Check sheet for the modelled part. Datum: model origin and axes. Units: mm. A direction names the side the tool comes from. Give positions to 0.01 mm unless a question says otherwise; leave off trailing zeros. Order: outer loops, then holes, each group sorted by start corner. A loop starts at its lowest first (then second) coordinate and runs counter-clockwise, first axis right, second up. Notation, with made-up numbers: (78.5, -18.75) -> (82.5, -18.75) arc R24 ccw to (82.5, -1.75) -> close; hole circle Ø8 at (28, 83.25). An arc over 180 degrees is marked (long way). Answer in a Markdown table with one row per item. Add a question column.
(1) Go/stop test with flat-tipped pins: pin 1 (1.5 mm diameter, centred on x = -1.5, z = -3.5, fed in from +Y); pin 2 (1 mm diameter, centred on x = 0.5, y = 1, fed in from -Z); pin 3 (0.6 mm diameter, centred on x = 3.5, z = 2, fed in from +Y); pin 4 (2 mm diameter, centred on x = 12, z = 10.5, fed in from -Y) (1 decimal). Record where each tip stops, or that it passes through.
(2) Cross-section at B-B (y = -2.5). Record the cut outline in (x, z) (1 decimal).
(3) Cross-section at A-A (x = -13). Record the cut outline in (y, z).
(4) Set-up check for faces 4 (the face through (-3.7, 1.295, 1.6)), 5 (the face through (16.66, 0.98, -0.11)): record each of +Z, -Z, +X, -X, +Y, -Y from which the full face is reachable in a straight line by a thin tool's end or side.
(5) Release check for a two-part mould opening along X. For faces 1 (the face through (1, -3.81, -3)), 2 (the face through (-2.8, 1.78, -2.8)), 3 (the face through (-11.182, 0.952, 2.915)) record: released by +X, released by -X, zero draft, split by the parting line, or undercut.
(6) Thickness scan on L1, parallel to Z at x = 0, y = 0.5; L2, parallel to Z at x = -7, y = 0.5; L3, parallel to X at y = -3.1, z = 0. Record the ranges inside material, lowest first. Write a range as [from, to].
```python
from build123d import *

# Parameters (mm, degrees)
EXTRUDE4_DEPTH          = 1.9304
SKETCH2_R               = 0.6604
CUT_EXTRUDE1_DEPTH      = 19.722050478
CIRPATTERN4_COUNT       = 6
SKETCH3_R               = 1.397
CUT_EXTRUDE2_DEPTH      = 12.7
CUT_EXTRUDE2_DEPTH_BACK = 12.7
SKETCH4_R               = 4.445
CUT_EXTRUDE3_DEPTH      = 0.635
SKETCH5_R               = 3.4925
SKETCH5_R_2             = 3.175
EXTRUDE5_DEPTH          = 1.143
RIB10_REACH             = 26.438
SKETCH8_WALL_W          = 52.220152264
SKETCH8_WALL_H          = 0.381
CIRPATTERN5_COUNT       = 8
SKETCH9_R               = 0.79375
CUT_EXTRUDE4_DEPTH      = 25.392925761
CIRPATTERN6_COUNT       = 6
SKETCH10_R              = 5.08
EXTRUDE6_DEPTH          = 0.762
FILLET2_R               = 0.508
SKETCH11_R              = 4.064
EXTRUDE7_DEPTH          = 3.048
FILLET3_R               = 0.889
SKETCH12_R              = 2.8575
CUT_EXTRUDE5_DEPTH      = 3.429
SKETCH14_R              = 1.397
CUT_EXTRUDE6_DEPTH      = 25.557003564
SKETCH15_R              = 0.3175
CUT_EXTRUDE7_DEPTH      = 25.984806887
CIRPATTERN7_COUNT       = 6


with BuildPart() as part:
    # Sketch1 → Extrude4 (new body)
    with BuildSketch(Plane(origin=(0, 0, 0), x_dir=(1, 0, 0), z_dir=(0, 1, 0))):
        with BuildLine():
            Line((5.775220615, -3.829827046), (0, 0))
            Line((0, 0), (5.775220615, 3.829827046))
            Line((5.775220615, 3.829827046), (6.35029977, 3.829827046))
            Line((6.35029977, 3.829827046), (6.35029977, 3.494998084))
            Line((6.35029977, 3.494998084), (15.87469147, 2.35207108))
            ThreePointArc((15.87469147, 2.35207108), (18.22419147, 0.00257108), (15.87469147, -2.34692892))
            Line((15.87469147, -2.34692892), (6.34969147, -3.48992892))
            Line((6.34969147, -3.48992892), (6.34969147, -3.829827046))
            Line((6.34969147, -3.829827046), (5.775220615, -3.829827046))
        make_face()
    extrude4 = extrude(amount=EXTRUDE4_DEPTH)

    # Sketch2 → Cut-Extrude1 (cut, through all)
    with BuildSketch(Plane(origin=(0, 1.9304, 0), x_dir=(-1, 0, 0), z_dir=(0, 1, 0))):
        with Locations((-6.342552501, -4.149920748)):
            Circle(SKETCH2_R)
        with Locations((-6.342552501, 4.149920748)):
            Circle(SKETCH2_R)
    extrude(amount=-CUT_EXTRUDE1_DEPTH, mode=Mode.SUBTRACT)

    # CirPattern4: Extrude4 ×6 about axis
    cirpattern4_axis = Axis((0, 0, 0), (0, 1, 0))
    for i in range(1, CIRPATTERN4_COUNT):
        add(extrude4.rotate(cirpattern4_axis, i * 360 / CIRPATTERN4_COUNT))

    # Sketch3 → Cut-Extrude2 (cut, two sides)
    with BuildSketch(Plane(origin=(0, 1.9304, 0), x_dir=(-1, 0, 0), z_dir=(0, 1, 0))) as cut_extrude2_sk:
        with Locations(Location((0, 0, 0), (0, 0, 90))):
            Circle(SKETCH3_R)
    extrude(amount=CUT_EXTRUDE2_DEPTH, mode=Mode.SUBTRACT)
    extrude(cut_extrude2_sk.sketch, amount=-CUT_EXTRUDE2_DEPTH_BACK, mode=Mode.SUBTRACT)

    # Sketch4 → Cut-Extrude3 (cut)
    with BuildSketch(Plane(origin=(0, 1.9304, 0), x_dir=(-1, 0, 0), z_dir=(0, 1, 0))):
        with Locations(Location((0, 0, 0), (0, 0, 90))):
            Circle(SKETCH4_R)
    extrude(amount=-CUT_EXTRUDE3_DEPTH, mode=Mode.SUBTRACT)

    # Sketch5 → Extrude5 (add)
    with BuildSketch(Plane(origin=(0, 1.2954, 0), x_dir=(-1, 0, 0), z_dir=(0, 1, 0))):
        Circle(SKETCH5_R)
        Circle(SKETCH5_R_2, mode=Mode.SUBTRACT)
    extrude(amount=EXTRUDE5_DEPTH)

    # Sketch8 wall → Rib10 (add, up to next)
    with BuildSketch(Plane(origin=(-3.967749561, 1.770078976, 0), x_dir=(-0.70753138537, -0.706681921883, 0), z_dir=(0.706681921883, -0.70753138537, 0)), mode=Mode.PRIVATE) as rib10_sk1:
        Rectangle(SKETCH8_WALL_W, SKETCH8_WALL_H)
    rib10_tool1 = extrude(rib10_sk1.sketch, amount=RIB10_REACH, mode=Mode.PRIVATE) - part.part
    rib10 = rib10_tool1.solids().sort_by_distance((-3.967749561, 1.770078976, 0))[0]
    add(rib10)

    # CirPattern5: Rib10 ×8 about axis
    cirpattern5_axis = Axis((0, 0, 0), (0, 1, 0))
    for i in range(1, CIRPATTERN5_COUNT):
        add(rib10.rotate(cirpattern5_axis, i * 360 / CIRPATTERN5_COUNT))

    # Sketch9 → Cut-Extrude4 (cut, through all)
    with BuildSketch(Plane(origin=(0, 1.9304, 0), x_dir=(-1, 0, 0), z_dir=(0, 1, 0))):
        with Locations(Location((7.935119114, 13.749171631, 0), (0, 0, 90))):
            Circle(SKETCH9_R)
        with Locations(Location((6.469197887, 11.209171631, 0), (0, 0, 90))):
            Circle(SKETCH9_R)
        with Locations(Location((5.00327666, 8.669171631, 0), (0, 0, 90))):
            Circle(SKETCH9_R)
    cut_extrude4 = extrude(amount=-CUT_EXTRUDE4_DEPTH, mode=Mode.SUBTRACT)

    # CirPattern6: Cut-Extrude4 ×6 about axis
    cirpattern6_axis = Axis((0, 0, 0), (0, 1, 0))
    for i in range(1, CIRPATTERN6_COUNT):
        add(cut_extrude4.rotate(cirpattern6_axis, i * 360 / CIRPATTERN6_COUNT), mode=Mode.SUBTRACT)

    # Sketch10 → Extrude6 (add)
    with BuildSketch(Plane.XZ):
        with Locations(Location((0, 0, 0), (0, 0, 90))):
            Circle(SKETCH10_R)
    extrude(amount=EXTRUDE6_DEPTH)

    # Fillet2
    fillet2_edges = [part.edges().sort_by_distance(p)[0] for p in [
        (0, 0, -5.08),
    ]]
    fillet(fillet2_edges, radius=FILLET2_R)

    # Sketch11 → Extrude7 (add)
    with BuildSketch(Plane.XZ.offset(0.762)):
        with Locations(Location((0, 0, 0), (0, 0, 90))):
            Circle(SKETCH11_R)
    extrude(amount=EXTRUDE7_DEPTH)

    # Fillet3
    fillet3_edges = [part.edges().sort_by_distance(p)[0] for p in [
        (0, -0.762, -4.064),
    ]]
    fillet(fillet3_edges, radius=FILLET3_R)

    # Sketch12 → Cut-Extrude5 (cut)
    with BuildSketch(Plane.XZ.offset(3.81)):
        with Locations(Location((0, 0, 0), (0, 0, 270))):
            Circle(SKETCH12_R)
    extrude(amount=-CUT_EXTRUDE5_DEPTH, mode=Mode.SUBTRACT)

    # Sketch14 → Cut-Extrude6 (cut, through all)
    with BuildSketch(Plane.XZ.offset(0.381)):
        with Locations(Location((0, 0, 0), (0, 0, 90))):
            Circle(SKETCH14_R)
    extrude(amount=-CUT_EXTRUDE6_DEPTH, mode=Mode.SUBTRACT)

    # Sketch15 → Cut-Extrude7 (cut, symmetric)
    with BuildSketch(Plane(origin=(0, 1.9304, 0), x_dir=(-1, 0, 0), z_dir=(0, 1, 0))):
        with Locations((-6.48724684, -3.751940905)):
            Circle(SKETCH15_R)
    cut_extrude7 = extrude(amount=CUT_EXTRUDE7_DEPTH, both=True, mode=Mode.SUBTRACT)

    # CirPattern7: Cut-Extrude7 ×6 about axis
    cirpattern7_axis = Axis((0, 0, 0), (0, 1, 0))
    for i in range(1, CIRPATTERN7_COUNT):
        add(cut_extrude7.rotate(cirpattern7_axis, i * 360 / CIRPATTERN7_COUNT), mode=Mode.SUBTRACT)


solid = part.part
```
Answer below:
| question | item | result |
|---|---|---|
| 1 | pin 1 | stops at y = 2.44 |
| 1 | pin 2 | stops at z = -8.38 |
| 1 | pin 3 | stops at y = 1.3 |
| 1 | pin 4 | passes through |
| 2 | outline | circle Ø8.1 at (0, 0); hole circle Ø5.7 at (0, 0) |
| 3 | outline | (0, -2.69) -> (1.93, -2.69) -> (1.93, -0.79) -> (0, -0.79) -> close; (0, 0.79) -> (1.93, 0.79) -> (1.93, 2.7) -> (0, 2.7) -> close |
| 4 | face 4 | +Y |
| 4 | face 5 | +Y, -Y |
| 5 | face 1 | zero draft |
| 5 | face 2 | undercut |
| 5 | face 3 | released by -X |
| 6 | L1 | z = [-7.18, -1.4], [1.4, 7.18] |
| 6 | L2 | z = [-15.9, -11.8], [-10.61, -5.62], [-3.41, 3.42], [5.63, 10.62], [11.8, 15.9] |
| 6 | L3 | x = [-4.06, -2.86], [2.86, 4.06] |
